from build123d import *

# Parameters (mm, degrees)
SKETCH2_W          = 60
SKETCH2_H          = 1
BASE_FLANGE1_DEPTH = 85
EDGE_FLANGE1_DEPTH = 85
EDGE_FLANGE2_DEPTH = 85
EDGE_FLANGE3_DEPTH = 60
EDGE_FLANGE4_DEPTH = 60
CUT_EXTRUDE4_DEPTH = 1
SKETCH20_W         = 10.5
SKETCH20_H         = 13.5
CUT_EXTRUDE5_DEPTH = 1
SKETCH21_R         = 1.7
CUT_EXTRUDE6_DEPTH = 109.687625791


# Sheet-metal steps are written as plain solids
with BuildPart() as part:
    # Sketch2 → Base-Flange1 (new body)
    with BuildSketch(Plane.XY):
        with Locations((30, -0.5)):
            Rectangle(SKETCH2_W, SKETCH2_H)
    extrude(amount=BASE_FLANGE1_DEPTH)

    # Edge-Flange1 section (across the edge) → Edge-Flange1 (add)
    with BuildSketch(Plane(origin=(61, 0, 85), x_dir=(-1, 0, 0), z_dir=(0, 0, -1))):
        with BuildLine():
            Line((-1, 1), (-1, 20))
            Line((-1, 20), (0, 20))
            Line((0, 20), (0, 1))
            ThreePointArc((0, 1), (0.292893219, 0.292893219), (1, 0))
            Line((1, 0), (1, -1))
            ThreePointArc((1, -1), (-0.414213562, -0.414213562), (-1, 1))
        make_face()
    extrude(amount=EDGE_FLANGE1_DEPTH)

    # Edge-Flange2 section (across the edge) → Edge-Flange2 (add)
    with BuildSketch(Plane(origin=(-1, 0, 0), x_dir=(1, 0, 0), z_dir=(0, 0, 1))):
        with BuildLine():
            Line((-1, 1), (-1, 20))
            Line((-1, 20), (0, 20))
            Line((0, 20), (0, 1))
            ThreePointArc((0, 1), (0.292893219, 0.292893219), (1, 0))
            Line((1, 0), (1, -1))
            ThreePointArc((1, -1), (-0.414213562, -0.414213562), (-1, 1))
        make_face()
    extrude(amount=EDGE_FLANGE2_DEPTH)

    # Edge-Flange3 section (across the edge) → Edge-Flange3 (add)
    with BuildSketch(Plane(origin=(0, 0, 86), x_dir=(0, 0, -1), z_dir=(1, 0, 0))):
        with BuildLine():
            Line((-1, 1), (-1, 20))
            Line((-1, 20), (0, 20))
            Line((0, 20), (0, 1))
            ThreePointArc((0, 1), (0.292893219, 0.292893219), (1, 0))
            Line((1, 0), (1, -1))
            ThreePointArc((1, -1), (-0.414213562, -0.414213562), (-1, 1))
        make_face()
    extrude(amount=EDGE_FLANGE3_DEPTH)

    # Edge-Flange4 section (across the edge) → Edge-Flange4 (add)
    with BuildSketch(Plane(origin=(60, 0, -1), x_dir=(0, 0, 1), z_dir=(-1, 0, 0))):
        with BuildLine():
            Line((-1, 1), (-1, 20))
            Line((-1, 20), (0, 20))
            Line((0, 20), (0, 1))
            ThreePointArc((0, 1), (0.292893219, 0.292893219), (1, 0))
            Line((1, 0), (1, -1))
            ThreePointArc((1, -1), (-0.414213562, -0.414213562), (-1, 1))
        make_face()
    extrude(amount=EDGE_FLANGE4_DEPTH)

    # Sketch19 → Cut-Extrude4 (cut)
    with BuildSketch(Plane.XY.offset(87)):
        with BuildLine():
            Line((47, 20), (47, 8))
            ThreePointArc((47, 8), (42, 3), (37, 8))
            Line((37, 8), (37, 20))
            Line((37, 20), (47, 20))
        make_face()
    extrude(amount=-CUT_EXTRUDE4_DEPTH, mode=Mode.SUBTRACT)

    # Sketch20 → Cut-Extrude5 (cut)
    with BuildSketch(Plane.XY.offset(-1)):
        with Locations((48.75, 13.25)):
            Rectangle(SKETCH20_W, SKETCH20_H)
    extrude(amount=-CUT_EXTRUDE5_DEPTH, mode=Mode.SUBTRACT)

    # Sketch21 → Cut-Extrude6 (cut, through all)
    with BuildSketch(Plane(origin=(0, 0, 0), x_dir=(1, 0, 0), z_dir=(0, 1, 0))):
        with Locations(Location((5.5, -5.5, 0), (0, 0, 270))):
            Circle(SKETCH21_R)
        with Locations(Location((54.5, -5.5, 0), (0, 0, 270))):
            Circle(SKETCH21_R)
        with Locations(Location((53, -79, 0), (0, 0, 270))):
            Circle(SKETCH21_R)
        with Locations(Location((7, -79, 0), (0, 0, 270))):
            Circle(SKETCH21_R)
    extrude(amount=-CUT_EXTRUDE6_DEPTH, mode=Mode.SUBTRACT)


solid = part.part
Geometry: final body of the model. Coordinates: model frame, mm. A direction names the side the tool comes from. Give positions to 0.01 mm unless a question says otherwise; leave off trailing zeros. Write each loop counter-clockwise with the first axis right and the second up, starting at its lowest first coordinate (ties: lowest second). Pieces come first, ordered by that corner, then holes.
(1) Cut plane A-A, the plane y = 10. Return loops of the section in (x, z), then the cut area to 4 significant figures.
(2) Cut plane B-B, the plane z = 79. Return loops of the section in (x, y), then the cut area to 3 significant figures.
(3) First-contact query: P1, Ø0.6, axis at x = -1.5, y = 10, coming from the -Z side; P2, Ø3, axis at x = 54.5, z = 5.5, coming from the -Y side; P3, Ø0.8, axis at y = 11.5, z = -1.5, coming from the +X side; P4, Ø1, axis at y = 9.5, z = 86, coming from the -X side. Flat tips, straight axial feed; report the tip coordinate or a pass-through.
(4) Ray query, line 1 (Z direction, x = 31, y = 3); line 2 (X direction, y = 18.25, z = 49); line 3 (X direction, y = -0.3, z = 79). Return the intervals inside material, ascending.
(5) Cut plane D-D, the plane x = 27. Return loops of the section in (y, z), then the cut area to 3 significant figures.
(6) Cut plane C-C, the plane z = 32. Return loops of the section in (x, y), then the cut area to 3 significant figures.
(7) Access query for faces 1 (the flat face through (61, 11, 43)), 2 (the cylindrical face through (55.65, -0.49, 4.25)), 3 (the flat face through (30, 11, -1)). Directions: +Z, -Z, +X, -X, +Y, -Y. A direction counts if a zero-diameter tool reaches every point of the face in a straight line with its end or side. Return the directions, or none.
(8) Mould query, pull axis Z, two halves, no side actions, for faces 4 (the flat face through (30, 11, 86)), 5 (the flat face through (-1.4, 9.6, 85)), 6 (the flat face through (30, 0, 42)), 7 (the flat face through (-1, 11, 42)). Classes: released by +Z, released by -Z, zero draft, split by the parting line, or undercut.
Values follow:
1. outline: (-2, 0) - (-1, 0) - (-1, 85) - (-2, 85) - close; (0, -2) - (43.5, -2) - (43.5, -1) - (0, -1) - close; (0, 86) - (37, 86) - (37, 87) - (0, 87) - close; (47, 86) - (60, 86) - (60, 87) - (47, 87) - close; (54, -2) - (60, -2) - (60, -1) - (54, -1) - close; (61, 0) - (62, 0) - (62, 85) - (61, 85) - close
1. area: 269.5 mm2
2. outline: (-2, 1) arc R2 ccw to (0, -1) - (5.3, -1) - (5.3, 0) - (0, 0) arc R1 cw to (-1, 1) - (-1, 20) - (-2, 20) - close; (8.7, -1) - (51.3, -1) - (51.3, 0) - (8.7, 0) - close; (54.7, -1) - (60, -1) arc R2 ccw to (62, 1) - (62, 20) - (61, 20) - (61, 1) arc R1 cw to (60, 0) - (54.7, 0) - close
2. area: 95.9 mm2
3. P1: stops at z = 0
3. P2: passes through
3. P3: stops at x = 60
3. P4: stops at x = 0
4. line 1: z = -2 to -1, 86 to 87
4. line 2: x = -2 to -1, 61 to 62
4. line 3: x = -1.52 to 5.3, 8.7 to 51.3, 54.7 to 61.52
5. outline: (-1, 0) arc R2 ccw to (1, -2) - (20, -2) - (20, -1) - (1, -1) arc R1 cw to (0, 0) - (0, 85) arc R1 cw to (1, 86) - (20, 86) - (20, 87) - (1, 87) arc R2 ccw to (-1, 85) - close
5. area: 128 mm2
6. outline: (-2, 1) arc R2 ccw to (0, -1) - (60, -1) arc R2 ccw to (62, 1) - (62, 20) - (61, 20) - (61, 1) arc R1 cw to (60, 0) - (0, 0) arc R1 cw to (-1, 1) - (-1, 20) - (-2, 20) - close
6. area: 103 mm2
7. face 1: +Z, -Z, +Y
7. face 2: +Y, -Y
7. face 3: +X, -X, +Y
8. face 4: undercut
8. face 5: released by +Z
8. face 6: undercut
8. face 7: zero draft
